Part model, mm, in its own coordinate system. A direction names the side the tool comes from. Round coordinates to 2 decimals unless told otherwise and drop trailing zeros. Loops run counter-clockwise (first coordinate to the right, second up) from the corner with the lowest first, then second, coordinate; pieces in that order, holes last. Notation, with made-up numbers: M 71.25,53 L 89.25,53 A23 cw 89.25,89 Z; hole C 13,22.25 d8. An arc over 180 degrees is marked long. Put each result on its own line as item: value. Start each with the question number.
1) Slice it at D-D on z = 6. Give the cut face in (x, y), then the cut area to 3 significant figures.
2) Probe line 1 along Y through (x, z) = (77.5, 13.5); line 2 along Z through (x, y) = (79, -1.2); line 3 along X through (y, z) = (0.95, -2.5). List the from-to ranges inside material, lowest first.
3) Drop flat-ended pins along their axis: pin 1 Ø2.5 at (x, z) = (67, -15.32) entering from -Y; pin 2 Ø3.5 at (x, z) = (55, -15.32) entering from -Y; pin 3 Ø1.5 at (y, z) = (1, -10.5) entering from +X; pin 4 Ø1.3 at (x, y) = (78, 0.5) entering from -Z. Give the stop position or say it passes through.
4) Which spindle directions (+Z, -Z, +X, -X, +Y, -Y) get a long thin tool onto all of the face, cutting with end or side? Do faces 4 (the cylindrical face through (74.5, -0.5, 23)), 5 (the flat face through (77, 0, 5)), 6 (the flat face through (61, 0, 3)). Say none if no direction does.
5) Slice it at B-B on z = 23. Give the cut face in (x, y), then the cut area to 3 significant figures.
6) Slice it at C-C on y = -0.9. Give the cut face in (x, z), then the cut area to 3 significant figures.
7) Pull direction Z, two halves, no side cores. Call faces 1 (the flat face through (52, 1, 22)), 2 (the flat face through (61, 2, -18.3)), 3 (the cylindrical face through (83.5, -0.5, 23)): +Z half, -Z half, draft (parallel to the pull), parting line (faces both ways), or undercut.
8) Slice it at A-A on x = 55. Give the cut face in (y, z), then the cut area to 3 significant figures.
Autodesk Inventor part; units mm, degrees
ref_plane "Work Plane1" through (65, 0, 65) normal (1, 0, 0) x (0, 0, -1)
ref_plane "Work Plane2" through (0, 0, 0) normal (0, 1, 0) x (-1, 0, 0)
ref_plane "Work Plane3" through (70, 0, 24.3197) normal (0, 0, 1) x (1, 0, 0)
sketch "Sketch1" plane through (0, 0, 0) normal (0, 1, 0) x (-1, 0, 0)
  line L0 (70, 0) -> (70, -70)
  line L1 (70, -70) -> (0, -70)
  line L2 (-70, 0) -> (-70, 70)
  line L3 (-70, 70) -> (0, 70)
  line L4 (0, 70) -> (70, 70)
  line L5 (70, 70) -> (70, 0)
  line L6 (0, -70) -> (-70, -70)
  line L7 (-70, -70) -> (-70, 0)
  point P0 (0, 0)
extrude "Extrusion1" add sketch "Sketch1" along normal blind 3
fillet "Fillet1" radius 5 3 edges at (70, 1.5, 70) (70, 1.5, -70) (-70, 1.5, 70)
fillet "Fillet2" radius 5 1 edges at (-70, 1.5, -70)
ref_plane "Work Plane1" through (65, 0, 65) normal (1, 0, 0) x (0, 0, -1)
sketch "Sketch6" plane through (70, 0, 65) normal (1, 0, 0) x (0, 0, -1)
  line L0 (65, 0) -> (57.2, 0)
  line L1 (130, 0) -> (0, 0)
  line L2 (65, 0) -> (72.8, 0)
  line L3 (57.2, 0) -> (57.2, -18)
  line L4 (72.8, 0) -> (72.8, -18)
  line L5 (65, 0) -> (65, -10)
  arc A0 (57.2, -18) -> (72.8, -18) centre (65, -10.2437) ccw
  line L6 (57.2, 0) -> (54.2, 0)
  line L7 (54.2, 0) -> (54.2, -18)
  line L8 (72.8, 0) -> (75.8, 0)
  line L9 (75.8, 0) -> (75.8, -18)
  arc A1 (54.2, -18) -> (75.8, -18) centre (65, -9.0916) ccw
  dimension "d17" = 18
  dimension "d21" = 3
  dimension "d22" = 3
extrude "Extrusion3" add sketch "Sketch6" against normal blind 18 contours L3 A0 L4 L1 L9 A1 L7
pattern_circular "Circular Pattern1" count 4 over 360 about axis through (0, -10, 0) along (0, 1, 0) of "Extrusion3"
sketch "Sketch8" plane through (0, 3, 0) normal (0, 1, 0) x (1, 0, 0)
  circle A0 centre (58.4636, -19.348) radius 2.5
  point P0 (0, 0)
  dimension "d35" = 5
extrude "Extrusion5" cut sketch "Sketch8" against normal blind 3
sketch "Sketch9" plane through (0, 3, 0) normal (0, 1, 0) x (1, 0, 0)
  circle A0 centre (-60.6489, 18.9578) radius 2.5
  point P0 (0, 0)
  dimension "d39" = 5
extrude "Extrusion6" cut sketch "Sketch9" against normal blind 3
sketch "Sketch10" plane through (0, 3, 0) normal (0, 1, 0) x (1, 0, 0)
  line L0 (70, -65) -> (70, 65)
  line L1 (70, 15.1257) -> (39.2687, 15.1257)
  line L2 (39.2687, 15.1257) -> (39.2687, -15.3197)
  line L3 (39.2687, -15.3197) -> (70, -15.3197)
  line L4 (70, -15.3197) -> (70, 15.1257)
  point P0 (0, 0)
extrude "Extrusion7" add sketch "Sketch10" along normal blind 10
sketch "Sketch12" plane through (0, 3, 0) normal (0, 1, 0) x (1, 0, 0)
  line L0 (39.2687, -15.3197) -> (39.2687, -70)
  line L1 (10.8, -70) -> (65, -70)
  line L2 (39.2687, -15.3197) -> (39.2687, 15.1257)
  line L3 (39.2687, -70) -> (-73.9803, -70)
  line L4 (-73.9803, -70) -> (-73.9803, 75.2408)
  line L5 (-73.9803, 75.2408) -> (39.2687, 75.2408)
  line L6 (39.2687, 75.2408) -> (39.2687, -70)
  point P0 (0, 0)
extrude "Extrusion8" cut sketch "Sketch12" against normal blind 100
sketch "Sketch13" plane through (0, 3, 0) normal (0, 1, 0) x (1, 0, 0)
  line L0 (39.2687, -15.3197) -> (74.5621, -15.3197)
  line L1 (74.5621, -15.3197) -> (74.5621, -76.2104)
  line L2 (74.5621, -76.2104) -> (39.2687, -76.2104)
  line L3 (39.2687, -76.2104) -> (39.2687, -15.3197)
  point P0 (0, 0)
extrude "Extrusion9" cut sketch "Sketch13" against normal blind 100
sketch "Sketch14" plane through (0, 3, 0) normal (0, 1, 0) x (1, 0, 0)
  line L0 (39.2687, 15.1257) -> (72.3919, 15.1257)
  line L1 (72.3919, 15.1257) -> (72.3919, 74.5163)
  line L2 (72.3919, 74.5163) -> (39.2687, 74.5163)
  line L3 (39.2687, 74.5163) -> (39.2687, 15.1257)
  point P0 (0, 0)
extrude "Extrusion10" cut sketch "Sketch14" against normal blind 100
sketch "Sketch17" plane through (70, -18, 10.8) normal (1, 0, 0) x (0, 0, -1)
  line L0 (-4.5197, 18) -> (-4.5197, 21)
  line L1 (-4.5197, 18) -> (-4.5197, 31)
  line L2 (-4.5197, 21) -> (25.9257, 21)
  line L3 (25.9257, 31) -> (25.9257, 18)
  line L4 (25.9257, 21) -> (-4.5197, 21)
  line L5 (-4.5197, 21) -> (-4.5197, 31)
  line L6 (-4.5197, 31) -> (25.9257, 31)
  line L7 (25.9257, 31) -> (25.9257, 21)
  point P0 (10.8, 18)
  dimension "d50" = 3
extrude "Extrusion11" cut sketch "Sketch17" against normal blind 100
sketch "Sketch18" plane through (39.2687, 0, -15.1257) normal (-1, 0, 0) x (0, 0, 1)
  line L0 (0, 3) -> (30.4454, 3)
  line L1 (30.4454, 3) -> (30.4454, 0)
  line L2 (30.4454, 0) -> (0, 0)
  line L3 (0, 0) -> (0, 3)
  point P0 (15.1257, 0)
extrude "Extrusion12" cut sketch "Sketch18" against normal blind 13
sketch "Sketch20" plane through (52, 0, 65) normal (-1, 0, 0) x (0, 0, 1)
  line L0 (-72.8, -18) -> (-72.8, 0)
  line L1 (-72.8, -9) -> (-57.2, -9)
  line L2 (-57.2, -18) -> (-57.2, 0)
  line L3 (-72.8, -18) -> (-72.8, -4)
  arc A0 (-72.8, -18) -> (-57.2, -18) centre (-65, -10.2437) ccw
  line L4 (-65, -21.2437) -> (-72.8, -21.2437)
  line L5 (-72.8, -4) -> (-72.8, -0.8)
  line L6 (-65, -21.2437) -> (-65, -3.2437)
  line L7 (-65, -21.2437) -> (-65, -11.2437)
  line L8 (-65, -11.2437) -> (-65, -1.2437)
  line L9 (-65, -1.2437) -> (-65, -0.8)
  arc A1 (-65, -0.8) -> (-72.6527, -4.1368) centre (-65, -11.2437) ccw
  arc A2 (-57.2, -4.2988) -> (-65, -0.8) centre (-65, -11.2437) ccw
  arc A3 (-72.6527, -4.1368) -> (-72.8, -4.2988) centre (-65, -11.2437) ccw
  arc A4 (-57.2, -4.2988) -> (-57.2, -4.2988) centre (-65, -11.2437) ccw
  line L10 (-72.8, -4.2988) -> (-72.8, 0)
  line L11 (-57.2, 0) -> (-57.2, -4.2988)
  line L12 (-57.2, 0) -> (-72.8, 0)
  line L13 (-57.2, -4.2988) -> (-57.2, 0)
  line L14 (-72.8, -4.2988) -> (-72.8, 0)
  line L15 (-72.8, 0) -> (-57.2, 0)
  point P0 (-65, 0)
  dimension "d55" = 14
  dimension "d56" = 3.2
  dimension "d57" = 18
  dimension "d58" = 10
  dimension "d59" = 10
extrude "Extrusion13" add sketch "Sketch20" against normal blind 18 contours L0 L12 L2 A2 A1 A3
sketch "Sketch22" plane through (52.2687, 0, 10.8) normal (0, 1, 0) x (1, 0, 0)
  line L0 (-0.2687, 21.6) -> (0, 21.6)
  line L1 (0, 21.6) -> (0, 0)
  line L2 (0, 0) -> (-0.2687, 0)
  line L3 (-0.2687, 0) -> (-0.2687, 21.6)
  point P0 (-52.2687, 10.8)
extrude "Extrusion14" add sketch "Sketch22" along normal blind 3
sketch "Sketch24" plane through (52.2687, 0, -15.1257) normal (-1, 0, 0) x (0, 0, 1)
  line L0 (30.4454, 3) -> (25.9257, 3)
  line L1 (25.9257, 3) -> (25.9257, 0)
  line L2 (25.9257, 0) -> (30.4454, 0)
  line L3 (30.4454, 0) -> (30.4454, 3)
  point P0 (15.1257, 0)
extrude "Extrusion16" add sketch "Sketch24" along normal blind 0.3
sketch "Sketch25" plane through (52.2687, 0, -15.1257) normal (-1, 0, 0) x (0, 0, 1)
  line L0 (0, 0) -> (4.3257, 0)
  line L1 (4.3257, 0) -> (4.3257, 3)
  line L2 (4.3257, 3) -> (0, 3)
  line L3 (0, 3) -> (0, 0)
  point P0 (15.1257, 0)
extrude "Extrusion17" add sketch "Sketch25" along normal blind 0.27
sketch "Sketch26" plane through (51.9687, 0, -15.1257) normal (-1, 0, 0) x (0, 0, 1)
  line L0 (30.4454, 3) -> (25.9257, 3)
  line L1 (25.9257, 3) -> (25.9257, 0)
  line L2 (25.9257, 0) -> (30.4454, 0)
  line L3 (30.4454, 0) -> (30.4454, 3)
  point P0 (15.1257, 0)
extrude "Extrusion18" cut sketch "Sketch26" against normal blind 0.03
sketch "Sketch27" plane through (70, 0, 15.3197) normal (0, 0, 1) x (1, 0, 0)
  line L0 (0, 3) -> (-18, 3)
  line L1 (-18, 3) -> (-18, 0)
  line L2 (-18, 0) -> (0, 0)
  line L3 (0, 0) -> (0, 3)
  point P0 (-70, 0)
extrude "Extrusion19" add sketch "Sketch27" along normal blind 3
sketch "Sketch32" plane through (51.9987, 0, -15.1257) normal (-1, 0, 0) x (0, 0, 1)
  line L0 (4.3257, 0) -> (-3, 0)
  line L1 (-3, 0) -> (-3, 3)
  line L2 (-3, 3) -> (4.3257, 3)
  line L3 (4.3257, 3) -> (4.3257, 0)
  point P0 (15.1257, 0)
extrude "Extrusion21" cut sketch "Sketch32" against normal blind 30
sketch "Sketch33" plane through (51.9987, 0, -15.1257) normal (-1, 0, 0) x (0, 0, 1)
  line L0 (33.4454, 0) -> (25.9257, 0)
  line L1 (25.9257, 3) -> (33.4257, 3)
  line L2 (33.4257, 3) -> (33.4257, 0)
  line L3 (33.4257, 0) -> (25.9257, 0)
  line L4 (25.9257, 0) -> (25.9257, 3)
  point P0 (15.1257, 0)
  dimension "d86" = 7.5
extrude "Extrusion22" add sketch "Sketch33" against normal blind 18
sketch "Sketch34" plane through (52, 3, -10.8) normal (0, 1, 0) x (1, 0, 0)
  line L0 (18, -29.1197) -> (18, -26.1197)
  line L1 (18, -29.1197) -> (18, -21.6)
  line L2 (18, -26.1197) -> (-0.0013, -26.1197)
  line L3 (-0.0013, -29.1) -> (-0.0013, -21.6)
  line L4 (-0.0013, -26.1197) -> (2.9987, -26.1197)
  line L5 (18, -26.1197) -> (15, -26.1197)
  circle A0 centre (15, -26.1197) radius 1.5
  circle A1 centre (2.9987, -26.1197) radius 1.5
  point P0 (-52, -10.8)
  dimension "d89" = 3
  dimension "d90" = 3
  dimension "d91" = 3
  dimension "d92" = 3
  dimension "d93" = 3
extrude "Extrusion23" cut sketch "Sketch34" against normal blind 18
sketch "Sketch35" plane through (70, -18, -10.8) normal (0, 0, -1) x (-1, 0, 0)
  line L0 (18, 21) -> (0, 21)
  line L1 (0, 21) -> (0, 18)
  line L2 (0, 18) -> (18, 18)
  line L3 (18, 18) -> (18, 21)
  point P0 (70, 18)
extrude "Extrusion24" add sketch "Sketch35" along normal blind 7.5
mirror "Mirror1" about plane through (0, 0, 0) normal (0, 0, 1) of "Extrusion23"
ref_plane "Work Plane2" through (0, 0, 0) normal (0, 1, 0) x (-1, 0, 0)
sketch "Sketch38" plane through (0, 0, 0) normal (0, 1, 0) x (-1, 0, 0)
  line L0 (-70, -18.3) -> (-51.9987, -18.3)
  line L1 (-51.9987, -18.3) -> (-51.9987, 18.3)
  line L2 (-51.9987, 18.3) -> (-70, 18.3)
  line L3 (-70, 18.3) -> (-70, -18.3)
  point P0 (0, 0)
extrude "Extrusion25" cut sketch "Sketch38" against normal blind 30
sketch "Sketch39" plane through (70, 0, 18.3197) normal (0, 0, 1) x (1, 0, 0)
  line L0 (0, 0) -> (-18, 0)
  line L1 (-18, 0) -> (-18, 3)
  line L2 (-18, 3) -> (0, 3)
  line L3 (0, 3) -> (0, 0)
  point P0 (-70, 0)
extrude "Extrusion26" add sketch "Sketch39" along normal blind 10
ref_plane "Work Plane3" through (70, 0, 24.3197) normal (0, 0, 1) x (1, 0, 0)
ref_plane "Work Plane4" through (70, 0, 14.3197) normal (0, 0, 1) x (1, 0, 0)
sketch "Sketch43" plane through (70, 0, 28.3197) normal (0, 0, 1) x (1, 0, 0)
  line L0 (0, 0) -> (-18, 0)
  line L1 (-18, 0) -> (-18, 3)
  line L2 (-18, 3) -> (0, 3)
  line L3 (0, 3) -> (0, 0)
  point P0 (-70, 0)
extrude "Extrusion27" cut sketch "Sketch43" against normal blind 3
sketch "Sketch44" plane through (70, 0, -18.3) normal (1, 0, 0) x (0, 0, -1)
  line L0 (-18.3, 0) -> (-23.3, 0)
  line L1 (-43.6197, 0) -> (0, 0)
  line L2 (-23.3, 0) -> (-43.6197, 0)
  line L3 (-43.6197, 0) -> (-43.6197, 3)
  line L4 (-43.6197, 3) -> (-23.3, 3)
  line L5 (-23.3, 3) -> (-23.3, 0)
  dimension "d116" = 5
ref_plane "Work Plane7" through (0, 0, 5) normal (0, 0, 1) x (1, 0, 0)
sketch "Sketch45" plane through (0, 0, 5) normal (0, 0, 1) x (1, 0, 0)
  line L0 (70, 3) -> (70, 1.5)
  line L1 (70, 1.5) -> (73, 1.5)
  line L2 (73, 1.5) -> (70, 3)
  line L3 (70, 0) -> (70, -1.5)
  line L4 (70, -1.5) -> (73, -1.5)
  line L5 (70, 0) -> (73, -1.5)
  line L6 (73, 0) -> (70, 1.5)
  point P0 (0, 0)
  dimension "d118" = 1.5
  dimension "d119" = 3
  dimension "d120" = 1.5
  dimension "d121" = 3
  dimension "d122" = 1.5
sweep "Sweep2" add profiles "Sketch44" path "Sketch45" path curves L6
sketch "Sketch46" plane through (73, -1.5, 5) normal (1, 0, 0) x (0, 0, -1)
  line L0 (-20.3197, 1.5) -> (-20.3197, 4.5)
  line L1 (0, 0) -> (-20.3197, 0)
  line L2 (-20.3197, 0) -> (-20.3197, 3)
  line L3 (-20.3197, 3) -> (0, 3)
  line L4 (0, 3) -> (0, 0)
  point P0 (5, 1.5)
extrude "Extrusion28" add sketch "Sketch46" along normal blind 12
sketch "Sketch47" plane through (73, -1.5, 5) normal (0, -1, 0) x (1, 0, 0)
  line L0 (12, 0) -> (12, 18)
  line L1 (12, 0) -> (12, 20.3197)
  line L2 (12, 18) -> (3, 18)
  arc A0 (3, 19.5) -> (3, 16.5) centre (3, 18) ccw
  line L3 (3, 16.5) -> (9, 16.5)
  line L4 (9, 16.5) -> (9, 18)
  arc A1 (9, 16.5) -> (9, 19.5) centre (9, 18) ccw
  line L5 (9, 19.5) -> (3, 19.5)
  point P0 (-73, -5)
  dimension "d127" = 18
  dimension "d128" = 9
  dimension "d129" = 1.5
  dimension "d130" = 6
extrude "Extrusion29" cut sketch "Sketch47" against normal blind 12
sketch "Sketch48" plane through (73, 1.5, 25.3197) normal (0, 1, 0) x (1, 0, 0)
  line L0 (12, 20.3197) -> (0, 20.3197)
  line L1 (0, 20.3197) -> (0, 0)
  line L2 (0, 0) -> (12, 0)
  line L3 (12, 0) -> (12, 20.3197)
  point P0 (-73, 25.3197)
extrude "Extrusion30" cut sketch "Sketch48" against normal blind 1
sketch "Sketch49" plane through (70, 0, 5) normal (0, 0, -1) x (-1, 0, 0)
  line L0 (0, 3) -> (-3, 0.5)
  line L1 (-3, 0.5) -> (-3, 1.5)
  line L2 (-3, 1.5) -> (-3, 0.5)
  line L3 (-3, 1.5) -> (0, 3)
  line L4 (0, 3) -> (-3, 1.5)
  point P0 (70, 0)
extrude "Extrusion31" cut sketch "Sketch49" against normal blind 25
properties part number "holder"
Recorded:
1. outline: M 52,0 L 70,0 L 73,-1.5 L 85,-1.5 L 85,0.5 L 73,0.5 L 70,3 L 52,3 Z
1. area: 85.5 mm2
2. line 1: y = -1.5 to 0.5
2. line 2: z = 5 to 21.5, 24.5 to 25.32
2. line 3: x = 52 to 70
3. pin 1: passes through
3. pin 2: stops at y = 0
3. pin 3: stops at x = 70
3. pin 4: stops at z = 5
4. face 4: +Y, -Y
4. face 5: -Z, +X, +Y, -Y
4. face 6: +Z, -Z, -X, -Y
5. outline: M 52,0 L 70,0 L 73,-1.5 L 74.5,-1.5 L 74.5,0.5 L 73,0.5 L 70,3 L 52,3 Z; M 83.5,-1.5 L 85,-1.5 L 85,0.5 L 83.5,0.5 Z
5. area: 67.5 mm2
6. outline: M 71.8,5 L 85,5 L 85,25.32 L 71.8,25.32 Z; hole M 76,21.5 L 82,21.5 A1.5 ccw 82,24.5 L 76,24.5 A1.5 ccw Z
6. area: 243 mm2
7. face 1: draft
7. face 2: -Z half
7. face 3: undercut
8. outline: M 0,-18.3 L 3,-18.3 L 3,-16.82 L 0,-16.82 Z; M 0,-13.82 L 3,-13.82 L 3,13.82 L 0,13.82 Z; M 0,16.82 L 3,16.82 L 3,25.32 L 0,25.32 Z
8. area: 113 mm2
